Could you check a few things on this model? Use its own coordinates, in mm. A direction names the side the tool comes from. Round coordinates to 2 decimals unless told otherwise and drop trailing zeros. Write each loop counter-clockwise with the first axis right and the second up, starting at its lowest first coordinate (ties: lowest second). Pieces come first, ordered by that corner, then holes. Notation, with made-up numbers: (28, 83) -> (43, 83) arc R22 ccw to (43, 103) -> close; hole circle Ø2 at (-6.75, 21). An arc over 180 degrees is marked (long way). One line per question, with ' | ' between items. Start each with the question number.
1. Imagine slicing it at A-A, the plane z = 0. List the corners of the cut face in (x, y) for me, and give its area (3 significant figures).
2. Imagine slicing it at C-C, the plane y = -3.75. List the corners of the cut face in (x, z) for me.
3. Thinking about a two-plate mould opening in Z: for faces 4 (the flat face through (4.6, -9, -2)), 5 (the cylindrical face through (2.268, -4.213, -10.161)), 6 (the cylindrical face through (1.18, 13.27, -2.1)), 7 (the cylindrical face through (2.268, 2.703, -8.584)), which applies, released by +Z, released by -Z, zero draft, split by the parting line, or undercut?
4. Imagine slicing it at B-B, the plane y = 0. List the corners of the cut face in (x, z) for me.
5. For faces 1 (the flat face through (1.14, -12.11, -2.25)), 2 (the flat face through (1.14, 12.11, 2.25)), 3 (the flat face through (1.14, -12.14, 2.25)), which set-ups out of +Z, -Z, +X, -X, +Y, -Y let a thin tool reach every point of the face, with its end or its side?
6. If I drill on line 1 along Z through (x, y) = (1.15, 0); line 2 along Y through (x, z) = (1.9, 0), over which ranges is the centre line in solid material (lowest first)? Write a range as [from, to].
7. For pin 1 Ø1.5 at (x, z) = (2.5, -4) entering from -Y; pin 2 Ø1.2 at (y, z) = (-12, 0.5) entering from +X; pin 3 Ø2 at (x, z) = (3.5, -2) entering from +Y; pin 4 Ø11 at (y, z) = (0, 0) entering from +X, each with a flat end and sliding along its axis, tell me the tip position at first contact or that it passes through.
from build123d import *

# Parameters (mm, degrees)
SKETCH1_R                     = 11
SKETCH1_R_2                   = 9
BOSS_EXTRUDE1_DEPTH           = 4.6
SKETCH1_3_R                   = 11
SKETCH1_3_R_2                 = 9
BOSS_EXTRUDE2_DEPTH           = 4.6
BOSS_EXTRUDE3_DEPTH           = 2.3
BOSS_EXTRUDE3_DRAFT           = -10
BOSS_EXTRUDE3_PROFILE_2_DEPTH = 2.3
BOSS_EXTRUDE3_PROFILE_2_DRAFT = -10
FILLET1_R                     = 0.5


with BuildPart() as part:
    # Sketch1 → Boss-Extrude1 (new body)
    with BuildSketch(Plane.YZ):
        with Locations(Location((0, 0, 0), (0, 0, 270))):
            Circle(SKETCH1_R)
        with Locations(Location((0, 0, 0), (0, 0, 270))):
            Circle(SKETCH1_R_2, mode=Mode.SUBTRACT)
    extrude(amount=BOSS_EXTRUDE1_DEPTH)

    # Sketch1_3 → Boss-Extrude2 (add)
    with BuildSketch(Plane.YZ):
        with Locations(Location((0, 0, 0), (0, 0, 270))):
            Circle(SKETCH1_3_R)
        with Locations(Location((0, 0, 0), (0, 0, 270))):
            Circle(SKETCH1_3_R_2, mode=Mode.SUBTRACT)
    extrude(amount=BOSS_EXTRUDE2_DEPTH)


with BuildPart() as boss_extrude3_tool:
    # Sketch2 → Boss-Extrude3 (with draft: the straight prism first)
    with BuildSketch(Plane(origin=(0, 0, 0), x_dir=(0, -1, 0), z_dir=(-1, 0, 0))):
        with BuildLine():
            Line((-13.623688731, -2.45), (-10.723688731, -2.45))
            Line((-10.723688731, -2.45), (-8.660109699, -2.45))
            ThreePointArc((-8.660109699, -2.45), (-9, 0), (-8.660109699, 2.45))
            Line((-8.660109699, 2.45), (-10.723688731, 2.45))
            Line((-10.723688731, 2.45), (-13.623688731, 2.45))
            Line((-13.623688731, 2.45), (-13.623688731, -2.45))
        make_face()
    extrude(amount=-BOSS_EXTRUDE3_DEPTH)
    # Boss-Extrude3: the draft: its side faces are tilted about the plane it starts from
    boss_extrude3_sides = [boss_extrude3_tool.faces().sort_by_distance(p)[0] for p in [
        (1.15, 11.141899215, -2.45),
        (1.15, 11.141899215, 2.45),
        (1.15, 9, 0),
        (1.15, 13.623688731, 0),
    ]]
    draft(boss_extrude3_sides, Plane(origin=(0, 0, 0), x_dir=(0, -1, 0), z_dir=(-1, 0, 0)), BOSS_EXTRUDE3_DRAFT)


with BuildPart() as part_1:
    add(part.part)

    # Boss-Extrude3: add boss_extrude3_tool
    add(boss_extrude3_tool.part)


with BuildPart() as boss_extrude3_profile_2_tool:
    # Sketch2 → Boss-Extrude3 profile 2 (with draft: the straight prism first)
    with BuildSketch(Plane(origin=(0, 0, 0), x_dir=(0, -1, 0), z_dir=(-1, 0, 0))):
        with BuildLine():
            Line((10.723688731, -2.45), (13.623688731, -2.45))
            Line((13.623688731, -2.45), (13.623688731, 2.45))
            Line((13.623688731, 2.45), (10.723688731, 2.45))
            Line((10.723688731, 2.45), (8.660109699, 2.45))
            ThreePointArc((8.660109699, 2.45), (9, 0), (8.660109699, -2.45))
            Line((8.660109699, -2.45), (10.723688731, -2.45))
        make_face()
    extrude(amount=-BOSS_EXTRUDE3_PROFILE_2_DEPTH)
    # Boss-Extrude3 profile 2: the draft: its side faces are tilted about the plane it starts from
    boss_extrude3_profile_2_sides = [boss_extrude3_profile_2_tool.faces().sort_by_distance(p)[0] for p in [
        (1.15, -11.141899215, -2.45),
        (1.15, -11.141899215, 2.45),
        (1.15, -13.623688731, 0),
        (1.15, -9, 0),
    ]]
    draft(boss_extrude3_profile_2_sides, Plane(origin=(0, 0, 0), x_dir=(0, -1, 0), z_dir=(-1, 0, 0)), BOSS_EXTRUDE3_PROFILE_2_DRAFT)


with BuildPart() as part_2:
    add(part_1.part)

    # Boss-Extrude3 profile 2: add boss_extrude3_profile_2_tool
    add(boss_extrude3_profile_2_tool.part)

    # Fillet1
    fillet1_edges = [part_2.edges().sort_by_distance(p)[0] for p in [
        (2.3, -11, 0),
        (2.3, 11, 0),
        (1.15, 13.420912703, 2.247223972),
        (2.3, 13.218136675, 0),
        (1.15, 13.420912703, -2.247223972),
        (1.149928959, 10.768004835, 2.247236499),
        (1.149928959, 10.768004835, -2.247236499),
        (1.15, -13.420912703, -2.247223972),
        (1.149928959, -10.768004835, -2.247236499),
        (1.149928959, -10.768004835, 2.247236499),
        (2.3, -13.218136675, 0),
        (1.15, -13.420912703, 2.247223972),
    ]]
    fillet(fillet1_edges, radius=FILLET1_R)


solid = part_2.part
Geometry results:
1) outline: (0, -13.62) -> (1.89, -13.29) arc R0.5 ccw to (2.3, -12.8) -> (2.3, -11.5) arc R0.5 cw to (2.8, -11) -> (4.6, -11) -> (4.6, -9) -> (0, -9) -> close; (0, 9) -> (4.6, 9) -> (4.6, 11) -> (2.8, 11) arc R0.5 cw to (2.3, 11.5) -> (2.3, 12.8) arc R0.5 ccw to (1.89, 13.29) -> (0, 13.62) -> close | area: 29.6 mm2
2) outline: (0, -10.34) -> (4.6, -10.34) -> (4.6, -8.18) -> (0, -8.18) -> close; (0, 8.18) -> (4.6, 8.18) -> (4.6, 10.34) -> (0, 10.34) -> close
3) face 4: zero draft | face 5: split by the parting line | face 6: released by -Z | face 7: undercut
4) outline: (0, -11) -> (4.6, -11) -> (4.6, -9) -> (0, -9) -> close; (0, 9) -> (4.6, 9) -> (4.6, 11) -> (0, 11) -> close
5) face 1: -Z, +X, -Y | face 2: +Z, +X, +Y | face 3: +Z, +X, -Y
6) line 1: z = [-11, -9], [9, 11] | line 2: y = [-13.29, -9], [9, 13.29]
7) pin 1: stops at y = -10.51 | pin 2: stops at x = 2.31 | pin 3: stops at y = 10.95 | pin 4: passes through
